```python
from build123d import *

# Parameters (mm, degrees)
BOSS_EXTRUDE1_DEPTH     = 139.7
SKETCH2_W               = 345.783161942
SKETCH2_H               = 1.27
CUT_EXTRUDE1_DEPTH      = 5.08
SKETCH3_W               = 134.62
SKETCH3_H               = 1.27
CUT_EXTRUDE2_DEPTH      = 5.08
SKETCH4_W               = 134.62
SKETCH4_H               = 1.27
CUT_EXTRUDE3_DEPTH      = 5.08
SKETCH5_W               = 76.2
SKETCH5_H               = 1.27
CUT_EXTRUDE4_DEPTH      = 5.08
CUT_EXTRUDE_THIN1_DEPTH = 2.54
SKETCH8_W               = 0.683613246
SKETCH8_H               = 35.161225601
SKETCH8_W_2             = 0.852269187
CUT_EXTRUDE5_DEPTH      = 2.54
SKETCH9_R               = 27.432823907
SKETCH9_R_2             = 24.892823907
CUT_EXTRUDE_THIN2_DEPTH = 2.54


with BuildPart() as part:
    # Sketch1 → Boss-Extrude1 (new body)
    with BuildSketch(Plane.XY):
        with BuildLine():
            Line((109.030585849, 26.343843493), (-58.952576093, 26.343843493))
            ThreePointArc((-58.952576093, 26.343843493), (-121.814368941, 0.30563634), (-147.852576093, -62.556156507))
            Line((-147.852576093, -62.556156507), (-147.852576093, -316.556156507))
            ThreePointArc((-147.852576093, -316.556156507), (-121.814368941, -379.417949355), (-58.952576093, -405.456156507))
            Line((-58.952576093, -405.456156507), (109.030585849, -405.456156507))
            ThreePointArc((109.030585849, -405.456156507), (171.892378697, -379.417949355), (197.930585849, -316.556156507))
            Line((197.930585849, -316.556156507), (197.930585849, -62.556156507))
            ThreePointArc((197.930585849, -62.556156507), (171.892378697, 0.30563634), (109.030585849, 26.343843493))
        make_face()
    extrude(amount=BOSS_EXTRUDE1_DEPTH)

    # Sketch2 → Cut-Extrude1 (cut)
    with BuildSketch(Plane.XY.offset(139.7)):
        with Locations((25.039004878, -63.191156507)):
            Rectangle(SKETCH2_W, SKETCH2_H)
    extrude(amount=-CUT_EXTRUDE1_DEPTH, mode=Mode.SUBTRACT)

    # Sketch3 → Cut-Extrude2 (cut)
    with BuildSketch(Plane.ZY.offset(147.852576093)):
        with Locations((67.31, -63.191156507)):
            Rectangle(SKETCH3_W, SKETCH3_H)
    extrude(amount=-CUT_EXTRUDE2_DEPTH, mode=Mode.SUBTRACT)

    # Sketch4 → Cut-Extrude3 (cut)
    with BuildSketch(Plane(origin=(197.930585849, 0, 0), x_dir=(0, 0, -1), z_dir=(1, 0, 0))):
        with Locations((-67.31, -63.191156507)):
            Rectangle(SKETCH4_W, SKETCH4_H)
    extrude(amount=-CUT_EXTRUDE3_DEPTH, mode=Mode.SUBTRACT)

    # Sketch5 → Cut-Extrude4 (cut)
    with BuildSketch(Plane(origin=(0, 0, 0), x_dir=(-1, 0, 0), z_dir=(0, 0, -1))):
        with Locations((-154.750585849, -63.191156507)):
            Rectangle(SKETCH5_W, SKETCH5_H)
        with Locations((104.672576093, -63.191156507)):
            Rectangle(SKETCH5_W, SKETCH5_H)
    extrude(amount=-CUT_EXTRUDE4_DEPTH, mode=Mode.SUBTRACT)

    # Sketch7 → Cut-Extrude-Thin1 (cut)
    with BuildSketch(Plane(origin=(0, 0, 0), x_dir=(-1, 0, 0), z_dir=(0, 0, -1))):
        with BuildLine():
            Line((80.517176093, -100.257382108), (-130.302823907, -100.257382108))
            ThreePointArc((-130.302823907, -100.257382108), (-141.079131252, -95.793689453), (-145.542823907, -85.017382108))
            Line((-145.542823907, -85.017382108), (-145.542823907, -63.826156507))
            Line((-145.542823907, -63.826156507), (-145.542823907, -60.016156507))
            Line((-145.542823907, -60.016156507), (95.757176093, -60.016156507))
            Line((95.757176093, -60.016156507), (95.757176093, -63.826156507))
            Line((95.757176093, -63.826156507), (95.757176093, -85.017382108))
            ThreePointArc((95.757176093, -85.017382108), (91.293483439, -95.793689453), (80.517176093, -100.257382108))
        make_face()
        with BuildLine():
            Line((80.517176093, -97.717382108), (-130.302823907, -97.717382108))
            ThreePointArc((-130.302823907, -97.717382108), (-139.283080028, -93.997638229), (-143.002823907, -85.017382108))
            Line((-143.002823907, -85.017382108), (-143.002823907, -63.826156507))
            Line((-143.002823907, -63.826156507), (-143.002823907, -62.556156507))
            Line((-143.002823907, -62.556156507), (93.217176093, -62.556156507))
            Line((93.217176093, -62.556156507), (93.217176093, -63.826156507))
            Line((93.217176093, -63.826156507), (93.217176093, -85.017382108))
            ThreePointArc((93.217176093, -85.017382108), (89.497432214, -93.997638229), (80.517176093, -97.717382108))
        make_face(mode=Mode.SUBTRACT)
    extrude(amount=-CUT_EXTRUDE_THIN1_DEPTH, mode=Mode.SUBTRACT)

    # Sketch8 → Cut-Extrude5 (cut)
    with BuildSketch(Plane(origin=(0, 0, 0), x_dir=(-1, 0, 0), z_dir=(0, 0, -1))):
        with Locations((-116.308779226, -80.136769308)):
            Rectangle(SKETCH8_W, SKETCH8_H)
        with Locations((66.1464415, -80.136769308)):
            Rectangle(SKETCH8_W_2, SKETCH8_H)
    extrude(amount=-CUT_EXTRUDE5_DEPTH, mode=Mode.SUBTRACT)

    # Sketch9 → Cut-Extrude-Thin2 (cut)
    with BuildSketch(Plane(origin=(0, 0, 0), x_dir=(-1, 0, 0), z_dir=(0, 0, -1))):
        with Locations((-24.892823907, -221.511266295)):
            Circle(SKETCH9_R)
        with Locations((-24.892823907, -221.511266295)):
            Circle(SKETCH9_R_2, mode=Mode.SUBTRACT)
    extrude(amount=-CUT_EXTRUDE_THIN2_DEPTH, mode=Mode.SUBTRACT)


solid = part.part
```
The model under review builds one solid part; all positions refer to its coordinate system, in mm. A direction names the side the tool comes from. Give positions to 0.01 mm unless a question says otherwise; leave off trailing zeros. Write each loop counter-clockwise with the first axis right and the second up, starting at its lowest first coordinate (ties: lowest second). Pieces come first, ordered by that corner, then holes. Notation, with made-up numbers: M 16.5,-36 L 50.5,-36 A21 cw 50.5,-27 Z; hole C -25,40 d7. An arc over 180 degrees is marked long. Write each question's results on one line, items separated by ' | '. Start each with the question number.
1. Mouldability with a two-part tool opening along Y and no side actions: class faces 1 (the flat face through (19, -246, 2.54)), 2 (the flat face through (25, -221, 0)), 3 (the cylindrical face through (172.58, -0.39, 68.87)) as released by +Y, released by -Y, zero draft, split by the parting line, or undercut.
2. For faces 4 (the cylindrical face through (171.2, -380.1, 68.9)), 5 (the flat face through (26, -63.826, 137)), 6 (the cylindrical face through (12.234, -245.849, 1.252)), list the 3-axis set-ups (+Z, -Z, +X, -X, +Y, -Y) from which the entire face can be reached by the end or side of a thin tool; tool diameter is ignored.
3. We need section B-B (x = -119.5). Write out the cut boundary in (y, z), and give its area (3 significant figures).
4. We need section C-C (y = -346). Write out the cut boundary in (x, z).
5. We need section A-A (z = 23.5). Write out the cut boundary in (x, y).
6. Insertion check: pin 1 Ø0.6 at (y, z) = (-63, 65) entering from -X; pin 2 Ø1.5 at (x, z) = (-101.5, 79.5) entering from +Y; pin 3 Ø2 at (x, z) = (-73.5, 1) entering from -Y. Each pin has a flat end and moves straight along its axis. Give the tip position at first contact, or say it passes through.
7. For probe 1 along X at (y, z) = (-320.5, 27); probe 2 along Y at (x, z) = (155, 54); probe 3 along Y at (x, z) = (122, 21), list the stretches that pass through material, from the lowest coordinate up. Write a range as [from, to].
8. We need section D-D (x = 167). Write out the cut boundary in (y, z).
Results found:
1) face 1: undercut | face 2: zero draft | face 3: released by +Y
2) face 4: +Z, -Z, +X, -Y | face 5: none | face 6: -Z
3) outline: M -381.65,0 L -63.83,0 L -63.83,5.08 L -62.56,5.08 L -62.56,0 L 2.54,0 L 2.54,139.7 L -62.56,139.7 L -62.56,134.62 L -63.83,134.62 L -63.83,139.7 L -381.65,139.7 Z | area: 53,700 mm^2
4) outline: M -142.84,0 L 192.91,0 L 192.91,139.7 L -142.84,139.7 Z
5) outline: M -147.85,-316.56 A88.9 ccw -58.95,-405.46 L 109.03,-405.46 A88.9 ccw 197.93,-316.56 L 197.93,-63.83 L 192.85,-63.83 L 192.85,-62.56 L 197.93,-62.56 A88.9 ccw 109.03,26.34 L -58.95,26.34 A88.9 ccw -147.85,-62.56 L -142.77,-62.56 L -142.77,-63.83 L -147.85,-63.83 Z
6) pin 1: stops at x = -142.77 | pin 2: stops at y = 15.91 | pin 3: stops at y = -404.42
7) probe 1: x = [-147.77, 197.84] | probe 2: y = [-392.65, 13.54] | probe 3: y = [-404.51, 25.39]
8) outline: M -383.96,0 L -63.83,0 L -63.83,5.08 L -62.56,5.08 L -62.56,0 L 4.84,0 L 4.84,139.7 L -62.56,139.7 L -62.56,134.62 L -63.83,134.62 L -63.83,139.7 L -383.96,139.7 Z
